Work out the finished part from the listing and answer in its coordinate system (mm). Coordinates: 2 decimals unless noted, no trailing zeros. Order: outer loops, then holes, each group sorted by start corner. A loop starts at its lowest first (then second) coordinate and runs counter-clockwise, first axis right, second up. Notation, with made-up numbers: (67, 49.5) -> (75, 49.5) arc R17 ccw to (75, 70.5) -> close; hole circle Ø4 at (-12.75, 5). An arc over 180 degrees is marked (long way). Write item = value, one per line. Start each with the question number.
Q1. Straight lines are drawn through the part: L1, parallel to Y at x = 0, z = -10.25; L2, parallel to Z at x = 2.25, y = 193.5 (3 decimals); L3, parallel to X at y = -292.1, z = 10.55. For each, find the intervals that lie inside material, in ascending order. Write a range as from..to.
Q2. The part is cut by section A-A, the plane y = 134. Determine the outline of the cut face in (x, z) (3 decimals).
Q3. A flat-ended cylindrical pin translates along its axis: pin 1 (6 mm diameter, centred on x = 0, y = -88.9, fed in from +Z). Find the tip coordinate at first contact, or state that the pin passes through.
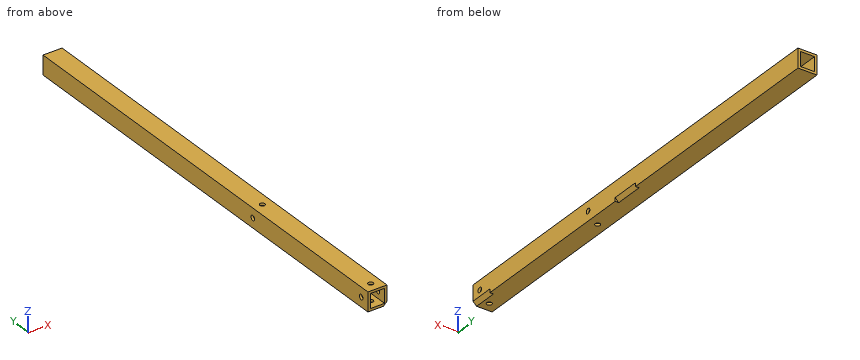
```python
from build123d import *

# Parameters (mm, degrees)
F0_W      = 25.4
F0_H      = 25.4
F0_W_2    = 19.05
F0_H_2    = 19.05
F1_DEPTH  = 304.8
F2_R      = 3.3782
F3_DEPTH  = 25.4
F4_R      = 3.3782
F5_DEPTH  = 25.4
F7_DEPTH  = 31.75
F10_DEPTH = 38.1


with BuildPart() as f1:
    # F0 (on Front) → F1 (new body, symmetric)
    with BuildSketch(Plane.XZ):
        Rectangle(F0_W, F0_H)
        Rectangle(F0_W_2, F0_H_2, mode=Mode.SUBTRACT)
    extrude(amount=F1_DEPTH, both=True)

    # F2 (on face) → F3 (cut, through all)
    with BuildSketch(Plane.XY.offset(12.7)):
        with Locations((0, -292.1)):
            Circle(F2_R)
        with Locations((0, -88.9)):
            Circle(F2_R)
    extrude(amount=-F3_DEPTH, mode=Mode.SUBTRACT)

    # F4 (on face) → F5 (cut, through all)
    with BuildSketch(Plane.YZ.offset(12.7)):
        with Locations((-292.1, 0)):
            Circle(F4_R)
        with Locations((-88.9, 0)):
            Circle(F4_R)
    extrude(amount=-F5_DEPTH, mode=Mode.SUBTRACT)

    # F6 (on face) → F7 (cut)
    with BuildSketch(Plane.XZ.offset(304.8)):
        Polygon((12.7, -12.7), (12.7, -7.9375), (7.9375, -12.7), align=None)
    extrude(amount=-F7_DEPTH, mode=Mode.SUBTRACT)

    # F9 (on offset) → F10 (cut)
    with BuildSketch(Plane.XZ.offset(38.1)):
        Polygon((12.7, -12.7), (12.7, -7.9375), (7.9375, -12.7), align=None)
    extrude(amount=-F10_DEPTH, mode=Mode.SUBTRACT)


solid = f1.part
```
Model answer:
q1.L1 = -304.8..-295.48, -288.72..-92.28, -85.52..304.8
q1.L2 = -12.7..-9.525, 9.525..12.7
q1.L3 = -12.7..-3.38, 3.38..12.7
q2.outline = (-12.7, -12.7) -> (12.7, -12.7) -> (12.7, 12.7) -> (-12.7, 12.7) -> close; hole (-9.525, -9.525) -> (9.525, -9.525) -> (9.525, 9.525) -> (-9.525, 9.525) -> close
q3.pin_1 = through
